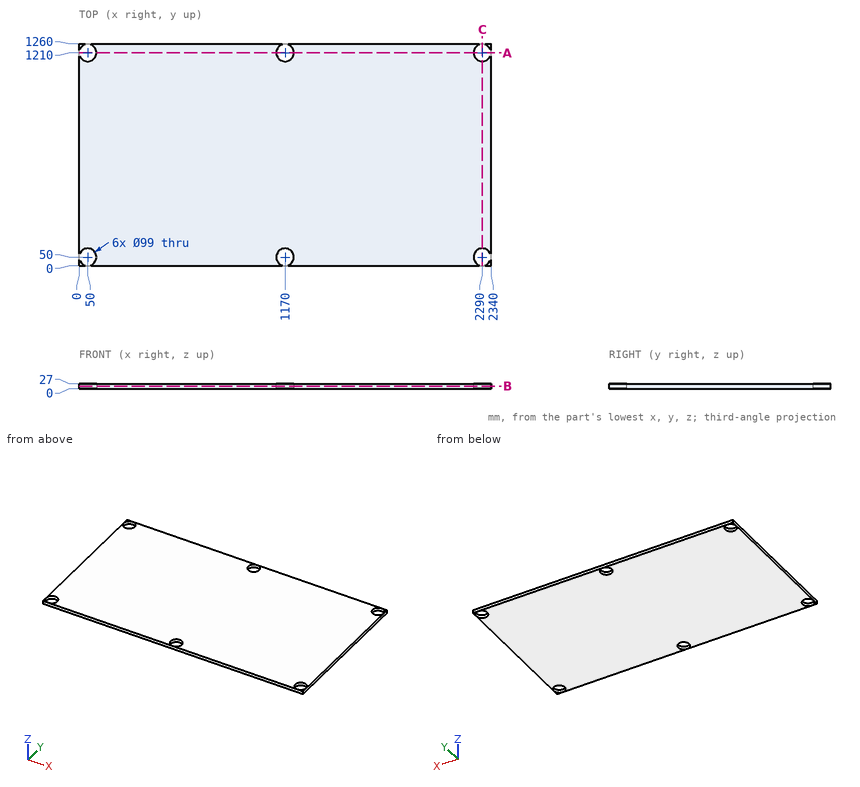
Design review of the part shown in the three views and the two pictorial views. Dimensions are in mm from the part's minimum x, y and z. Give positions to 0.01 mm unless a question says otherwise; leave off trailing zeros. Write each loop counter-clockwise with the first axis right and the second up, starting at its lowest first coordinate (ties: lowest second). Pieces come first, ordered by that corner, then holes. Notation, with made-up numbers: M -8.75,73 L 21.25,73 A13 ccw 21.25,98 Z; hole C -37.5,38.25 d5. An arc over 180 degrees is marked long. Return JSON: item names as keys, results as strings. Group by question number.
Item 1: Wall thickness on line 1 along Y through (x, z) = (2290, 14); line 2 along Y through (x, z) = (1166.5, 7); line 3 along X through (y, z) = (86.5, 18.25): over which ranges is each line inside the solid? List them lowest first.
Item 2: Take a section at C-C (x = 2290). Give the boundary of the cut face in (y, z), plus the area to 3 significant figures.
Item 3: Take a section at B-B (z = 14.5). Give the boundary of the cut face in (x, y).
Item 4: Take a section at A-A (y = 1210). Give the boundary of the cut face in (x, z), plus the area to 3 significant figures.
Return value:
{
 "1": {"line 1": "y = 0 to 0.5, 99.5 to 1160.5, 1259.5 to 1260", "line 2": "y = 0 to 0.62, 99.38 to 1160.62, 1259.38 to 1260", "line 3": "x = 0 to 16.56, 83.44 to 1136.56, 1203.44 to 2256.56, 2323.44 to 2340"},
 "2": {"outline": "M 0,0 L 0.5,0 L 0.5,27 L 0,27 Z; M 99.5,0 L 1160.5,0 L 1160.5,27 L 99.5,27 Z; M 1259.5,0 L 1260,0 L 1260,27 L 1259.5,27 Z", "area": "28,700 mm2"},
 "3": {"outline": "M 0,0 L 2340,0 L 2340,1260 L 0,1260 Z; hole C 50,50 d99; hole C 50,1210 d99; hole C 1170,50 d99; hole C 1170,1210 d99; hole C 2290,50 d99; hole C 2290,1210 d99"},
 "4": {"outline": "M 0,0 L 0.5,0 L 0.5,27 L 0,27 Z; M 99.5,0 L 1120.5,0 L 1120.5,27 L 99.5,27 Z; M 1219.5,0 L 2240.5,0 L 2240.5,27 L 1219.5,27 Z; M 2339.5,0 L 2340,0 L 2340,27 L 2339.5,27 Z", "area": "55,200 mm2"}
}
